Here's how the part is built. I have some questions about the finished solid (model axes, mm). A direction names the side the tool comes from. Round coordinates to 2 decimals unless told otherwise and drop trailing zeros. Loops run counter-clockwise (first coordinate to the right, second up) from the corner with the lowest first, then second, coordinate; pieces in that order, holes last. Notation, with made-up numbers: (85, 68) - (96, 68) arc R21 ccw to (96, 72) - close; hole circle Ø11 at (69.5, -9.5). An arc over 180 degrees is marked (long way). Return JSON: item names as keys, results as strings. Group by question number.
```python
from build123d import *

# Parameters (mm, degrees)
SKETCH1_W           = 42.3
SKETCH1_H           = 42.3
BOSS_EXTRUDE1_DEPTH = 48
CHAMFER1_SIZE       = 5
SKETCH3_R           = 1.5
CUT_EXTRUDE1_DEPTH  = 5
SKETCH4_R           = 11
BOSS_EXTRUDE2_DEPTH = 2
SKETCH5_R           = 2.5
BOSS_EXTRUDE3_DEPTH = 23
SKETCH6_W           = 16
SKETCH6_H           = 7
BOSS_EXTRUDE4_DEPTH = 9.6


with BuildPart() as part:
    # Sketch1 → Boss-Extrude1 (new body)
    with BuildSketch(Plane.XY):
        Rectangle(SKETCH1_W, SKETCH1_H)
    extrude(amount=-BOSS_EXTRUDE1_DEPTH)

    # Chamfer1
    chamfer1_edges = [part.edges().sort_by_distance(p)[0] for p in [
        (21.15, -21.15, -24),
        (-21.15, -21.15, -24),
        (-21.15, 21.15, -24),
        (21.15, 21.15, -24),
    ]]
    chamfer(chamfer1_edges, length=CHAMFER1_SIZE)

    # Sketch3 → Cut-Extrude1 (cut)
    with BuildSketch(Plane.XY):
        with Locations((15.5, -15.5)):
            Circle(SKETCH3_R)
        with Locations((-15.5, -15.5)):
            Circle(SKETCH3_R)
        with Locations((-15.5, 15.5)):
            Circle(SKETCH3_R)
        with Locations((15.5, 15.5)):
            Circle(SKETCH3_R)
    extrude(amount=-CUT_EXTRUDE1_DEPTH, mode=Mode.SUBTRACT)

    # Sketch4 → Boss-Extrude2 (add)
    with BuildSketch(Plane.XY):
        Circle(SKETCH4_R)
    extrude(amount=BOSS_EXTRUDE2_DEPTH)

    # Sketch5 → Boss-Extrude3 (add)
    with BuildSketch(Plane.XY):
        Circle(SKETCH5_R)
    extrude(amount=BOSS_EXTRUDE3_DEPTH)

    # Sketch6 → Boss-Extrude4 (add)
    with BuildSketch(Plane(origin=(0, 0, -48), x_dir=(-1, 0, 0), z_dir=(0, 0, -1))):
        with Locations((0, -24.65)):
            Rectangle(SKETCH6_W, SKETCH6_H)
    extrude(amount=-BOSS_EXTRUDE4_DEPTH)


solid = part.part
```
Q1. For faces 5 (the flat face through (0, 21.15, -24)), 6 (the flat face through (-8, -25, -43)), 7 (the cylindrical face through (14, -15.43, -2.46)), 8 (the flat face through (21.15, 0, -24)), 9 (the flat face through (0, -25, -38.4)), which set-ups out of +Z, -Z, +X, -X, +Y, -Y let a thin tool reach every point of the face, with its end or its side?
Q2. Imagine slicing it at A-A, the plane z = -42.5. List the corners of the cut face in (x, y) for me, and give its area (3 significant figures).
Q3. Please list where these lines run through material, in increasing order: line 1 (Y direction, x = -15.5, z = -2.5); line 2 (Y direction, x = -15, z = -3); line 3 (Z direction, x = 19.5, y = 2.5).
Q4. Imagine slicing it at D-D, the plane y = 10. List the corners of the cut face in (x, z) for me, and give its area (3 significant figures).
Q5. Imagine slicing it at B-B, the plane y = 0. List the corners of the cut face in (x, z) for me, and give its area (3 significant figures).
Q6. If we mould it in two halves opening along Y, with no side actions, what happens to faces 1 (the cylindrical face through (-2.38, -10.74, 0.99)), 2 (the flat face through (0, -28.15, -43)), 3 (the flat face through (-16, 16, -5)), 4 (the flat face through (-16, -15, -5))? For each: +Y half, -Y half, draft (parallel to the pull), parting line (faces both ways), or undercut.
Q7. Will these pins go through, and if not, where does the flat tip stop? pin 1 Ø5 at (x, y) = (0.5, 10) entering from +Z; pin 2 Ø3.5 at (y, z) = (-24.5, -44) entering from +X; pin 3 Ø5 at (x, y) = (-15.5, -15.5) entering from +Z; pin 4 Ø1 at (x, z) = (-3.5, 10.5) entering from -Y.
Q8. Imagine slicing it at C-C, the plane z = -30.5. List the corners of the cut face in (x, y) for me.
Output values:
{
 "1": {"face 5": "+Z, -Z, +X, -X, +Y", "face 6": "+Z, -Z, -X, -Y", "face 7": "+Z", "face 8": "+Z, -Z, +X, +Y, -Y", "face 9": "+Z, +X, -X, -Y"},
 "2": {"outline": "(-21.15, -16.15) - (-16.15, -21.15) - (-8, -21.15) - (-8, -28.15) - (8, -28.15) - (8, -21.15) - (16.15, -21.15) - (21.15, -16.15) - (21.15, 16.15) - (16.15, 21.15) - (-16.15, 21.15) - (-21.15, 16.15) - close", "area": "1,850 mm^2"},
 "3": {"line 1": "y = -21.15 to -17, -14 to 14, 17 to 21.15", "line 2": "y = -21.15 to -16.91, -14.09 to 14.09, 16.91 to 21.15", "line 3": "z = -48 to 0"},
 "4": {"outline": "(-21.15, -48) - (21.15, -48) - (21.15, 0) - (4.58, 0) - (4.58, 2) - (-4.58, 2) - (-4.58, 0) - (-21.15, 0) - close", "area": "2,050 mm^2"},
 "5": {"outline": "(-21.15, -48) - (21.15, -48) - (21.15, 0) - (11, 0) - (11, 2) - (2.5, 2) - (2.5, 23) - (-2.5, 23) - (-2.5, 2) - (-11, 2) - (-11, 0) - (-21.15, 0) - close", "area": "2,180 mm^2"},
 "6": {"face 1": "parting line", "face 2": "-Y half", "face 3": "undercut", "face 4": "undercut"},
 "7": {"pin 1": "stops at z = 2", "pin 2": "stops at x = 8", "pin 3": "stops at z = 0", "pin 4": "passes through"},
 "8": {"outline": "(-21.15, -16.15) - (-16.15, -21.15) - (16.15, -21.15) - (21.15, -16.15) - (21.15, 16.15) - (16.15, 21.15) - (-16.15, 21.15) - (-21.15, 16.15) - close"}
}
